Solid Edge part; units mm, degrees
sketch "Sketch1" plane through (0, 0, 0) normal (0, 0, 1) x (1, 0, 0)
  line L0 (-42, -50) -> (42, -50)
  line L1 (50, -42) -> (50, 42)
  line L2 (42, 50) -> (-42, 50)
  line L3 (-50, 42) -> (-50, -42)
  arc A0 (50, -42) -> (42, -50) centre (50, -50) cw
  arc A1 (42, 50) -> (50, 42) centre (50, 50) cw
  arc A2 (-50, 42) -> (-42, 50) centre (-50, 50) cw
  arc A3 (-42, -50) -> (-50, -42) centre (-50, -50) cw
extrude "Protrusion1" add sketch "Sketch1" along normal blind 2
shell "Thinwall_3" thickness 0.5 removed faces 1 at (-39.8267, -37.5067, 2)
sketch "Sketch2" plane through (0, 0, 0) normal (0, 0, 1) x (1, 0, 0)
  line L0 (-50, 42) -> (-50, -42)
  line L1 (42, 50) -> (-42, 50)
  line L2 (50, -42) -> (50, 42)
  line L3 (-42, -50) -> (42, -50)
  arc A0 (-42, -50) -> (-50, -42) centre (-50, -50) cw
  arc A1 (-50, 42) -> (-42, 50) centre (-50, 50) cw
  arc A2 (42, 50) -> (50, 42) centre (50, 50) cw
  arc A3 (50, -42) -> (42, -50) centre (50, -50) cw
extrude "ExtrudedProtrusion_6" add sketch "Sketch2" against normal blind 6.3715
sketch "Sketch3" plane through (0, 0, 0.5) normal (0, 0, 1) x (1, 0, 0)
  line L0 (-30, -30) -> (30, -30)
  line L1 (30, -30) -> (30, 30)
  line L2 (30, 30) -> (-30, 30)
  line L3 (-30, 30) -> (-30, -30)
extrude "ExtrudedProtrusion_7" add sketch "Sketch3" along normal blind 32
chamfer "Chamfer_2" distance 7 angle 45 4 edges at (-30, -30, 16.5) (30, -30, 16.5) (-30, 30, 16.5) (30, 30, 16.5)
sketch "Sketch4" plane through (0, 0, 0) normal (0, -1, 0) x (1, 0, 0)
  line L0 (0, 32.5) -> (12.5531, 32.5)
  line L1 (0, 32.5) -> (0, 36.5152)
  line L2 (0, 36.5152) -> (0, 49.6949)
  arc A0 (0, 49.6949) -> (12.5532, 32.5) centre (0, 36.5152) cw
revolve "RevolvedProtrusion1" add sketch "Sketch4" angle 360 about axis through (0, 0, 36.5152) along (0, 0, 1)
sketch "Sketch5" plane through (0, 0, -6.3715) normal (0, 0, -1) x (1, 0, 0)
  circle A0 centre (-30, 23) radius 0.75
  circle A1 centre (-23, 30) radius 0.75
  circle A2 centre (23, 30) radius 0.75
  circle A3 centre (30, 23) radius 0.75
  circle A4 centre (30, -23) radius 0.75
  circle A5 centre (23, -30) radius 0.75
  circle A6 centre (-30, -23) radius 0.75
  circle A7 centre (-23, -30) radius 0.75
extrude "ExtrudedProtrusion_10" add sketch "Sketch5" against normal blind 43.2945
sketch "Sketch6" plane through (0, -30, 16.5) normal (0, -1, 0) x (1, 0, 0)
  line L0 (16, 17) -> (-16, 17)
  line L1 (-16, 17) -> (-16, -16)
  line L2 (-16, -16) -> (0, -16)
  line L3 (0, -16) -> (16, -16)
  line L4 (16, -16) -> (16, 17)
extrude "ExtrudedProtrusion_11" add sketch "Sketch6" along normal blind 1
sketch "Sketch7" plane through (0, -31, 17) normal (0, -1, 0) x (1, 0, 0)
  line L0 (-10.3485, -13.2862) -> (-10.3485, 11.2862)
  line L1 (-10.3485, 11.2862) -> (10.3398, 11.2862)
  line L2 (10.3398, 11.2862) -> (10.3398, -13.2862)
  line L3 (10.3398, -13.2862) -> (-10.3485, -13.2862)
  line L4 (13.0457, 14.5) -> (-13.0543, 14.5)
  line L5 (-13.0543, 14.5) -> (-13.0543, -16.5)
  line L6 (-13.0543, -16.5) -> (13.0457, -16.5)
  line L7 (13.0457, -16.5) -> (13.0457, 14.5)
extrude "Protrusion2" add sketch "Sketch7" along normal blind 0.01
Source: CAD feature listing. Evaluate the final solid. Frame: model axes, mm. A direction names the side the tool comes from. Give positions to 0.01 mm unless a question says otherwise; leave off trailing zeros. Loops run counter-clockwise (first coordinate to the right, second up) from the corner with the lowest first, then second, coordinate; pieces in that order, holes last. Notation, with made-up numbers: (83.25, -6) - (128.25, -6) arc R10 cw to (128.25, 5) - close; hole circle Ø8 at (86, -14.5). An arc over 180 degrees is marked (long way). Use CSV: the item, a comma, the result in double quotes.
1) Pin query (flat end, axial travel): P1, Ø1.2, axis at y = 3.5, z = 1, coming from the -X side; P2, Ø3, axis at x = 31, y = -1.5, coming from the +Z side; P3, Ø1.5, axis at x = 5.5, z = 41, coming from the -Y side. Return the tip coordinate at first contact, or that it passes through.
Worked out:
P1,"stops at x = -50"
P2,"stops at z = 32.5"
P3,"stops at y = -11.55"
2) Cut plane D-D (y = -47). Output: boundary loops of the cut face in (x, z), and give its area (3 significant figures).
Worked out:
outline,"(-57.42, -6.37) - (57.42, -6.37) - (57.42, 2) - (56.87, 2) - (56.87, 0.5) - (-56.87, 0.5) - (-56.87, 2) - (-57.42, 2) - close"
area,"791 mm^2"
3) Line query: line 1 (Z direction, x = -15.5, y = -47); line 2 (Y direction, x = 20.5, z = 15). Output: solid intervals per line, ascending.
Worked out:
line 1,"z = -6.37 to 0.5"
line 2,"y = -30 to 30"
4) Set-up query: faces 4 (the flat face through (1, 50, -2)), 5 (the flat face through (-1, -50, -2)), 6 (the flat face through (-34, 9, 0.5)). Return all of +Z, -Z, +X, -X, +Y, -Y with unobstructed straight access to the full face (end or side cutting, diameter ignored); none if empty.
Worked out:
face 4,"+Z, -Z, +Y"
face 5,"+Z, -Z, -Y"
face 6,"+Z"
5) Cut plane A-A (y = 27.5). Output: boundary loops of the cut face in (x, z).
Worked out:
outline,"(-50, -6.37) - (50, -6.37) - (50, 2) - (49.5, 2) - (49.5, 0.5) - (25.5, 0.5) - (25.5, 32.5) - (-25.5, 32.5) - (-25.5, 0.5) - (-49.5, 0.5) - (-49.5, 2) - (-50, 2) - close"
6) Cut plane C-C (y = -35). Output: boundary loops of the cut face in (x, z).
Worked out:
outline,"(-50, -6.37) - (50, -6.37) - (50, 2) - (49.5, 2) - (49.5, 0.5) - (-49.5, 0.5) - (-49.5, 2) - (-50, 2) - close"
7) Mould query, pull axis X, two halves, no side actions, for faces 1 (the flat face through (0, -31, 16)), 2 (the flat face through (50, -1, -2)), 3 (the cylindrical face through (55.1, 55.5, 1.2)). Classes: +X half, -X half, draft (parallel to the pull), parting line (faces both ways), or undercut.
Worked out:
face 1,"draft"
face 2,"+X half"
face 3,"undercut"
